Answer from the drawing. Dimensions are ordinates in mm from the lowest x, y and z of the part. A direction names the side the tool comes from. Coordinates: 2 decimals unless noted, no trailing zeros. Write each loop counter-clockwise with the first axis right and the second up, starting at its lowest first coordinate (ties: lowest second). Pieces come first, ordered by that corner, then holes. Notation, with made-up numbers: (59, 64.25) -> (93, 64.25) arc R31 ccw to (93, 97.25) -> close; hole circle Ø5 at (12, 49.5). An arc over 180 degrees is marked (long way). One line per item, written item: value. Start each with the question number.
1. Consider line 1 along Y through (x, z) = (14, 6); line 2 along Z through (x, y) = (69, 15.5); line 3 along Z through (x, y) = (44.5, 2.25). Determine where each line is inside the solid, lowest interval first.
2. Find section A-A, the plane x = 99. Write down the section's boundary in (y, z).
3. Given P1, Ø2, axis at y = 15.5, z = 5.5, coming from the +X side, flat-ended and moving along its own axis, determine where the tip first touches the part or whether it passes through.
4. Find section B-B, the plane y = 16. Write down the section's boundary in (x, z).
5. For the marked faces 1 and 2, determine the directions among +Z, -Z, +X, -X, +Y, -Y from which every point of the face is accessible in a straight line to the end or side of a thin tool.
6. Find section C-C, the plane y = 2. Write down the section's boundary in (x, z), and give its area (3 significant figures).
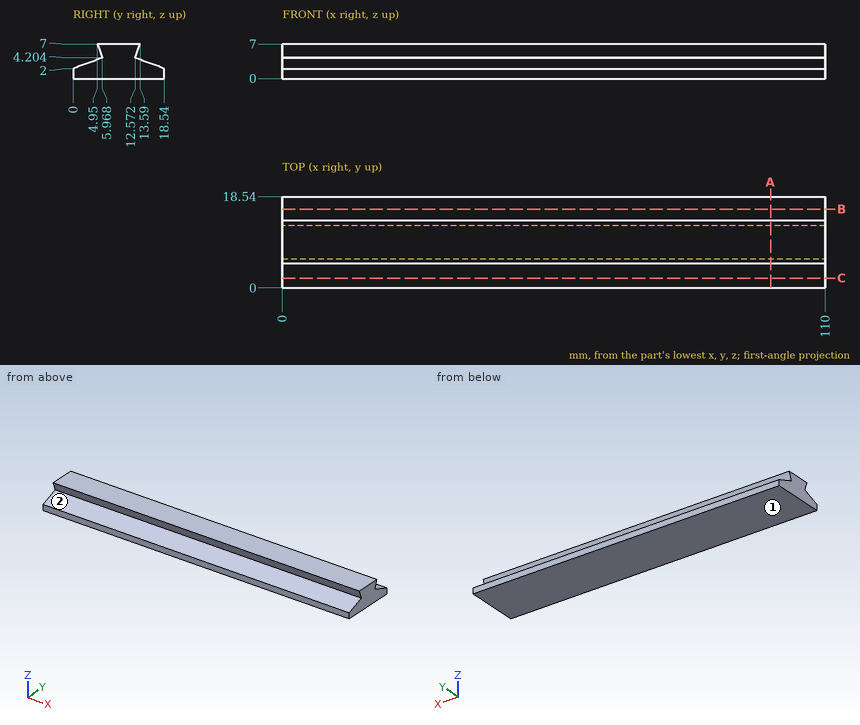
Answer block:
1. line 1: y = 5.31 to 13.23
1. line 2: z = 0 to 3.12
1. line 3: z = 0 to 2.83
2. outline: (0, 0) -> (18.54, 0) -> (18.54, 2) -> (12.57, 4.2) -> (13.59, 7) -> (4.95, 7) -> (5.97, 4.2) -> (0, 2) -> close
3. P1: passes through
4. outline: (0, 0) -> (110, 0) -> (110, 2.94) -> (0, 2.94) -> close
5. face 1: -Z, +X, -X, +Y, -Y
5. face 2: +X, -X, -Y
6. outline: (0, 0) -> (110, 0) -> (110, 2.74) -> (0, 2.74) -> close
6. area: 301 mm2
